Read the model definition and answer for the solid it produces. Units are mm, in the model's axes. Face numbers are marked on the shaded views. A direction names the side the tool comes from. Round coordinates to 2 decimals unless told otherwise and drop trailing zeros. Order: outer loops, then holes, each group sorted by start corner. A loop starts at its lowest first (then second) coordinate and runs counter-clockwise, first axis right, second up. Notation, with made-up numbers: (9.5, 13) - (27.5, 13) arc R21 ccw to (27.5, 41) - close; hole circle Ø8 at (-8.75, 4.5). An arc over 180 degrees is marked (long way). Put each result on its own line as item: value. Start each with the question number.
Q1. Which of the six approach directions +Z, -Z, +X, -X, +Y, -Y give full straight-line access (tool end or side, diameter ignored) to the marked faces 3 and 4?
Q2. Find the intervals of material crossed by line 1 along Y through (x, z) = (2.3, 28.5); line 2 along X through (y, z) = (0.75, 5.5); line 3 along Y through (x, z) = (1.65, 30), in increasing order. Write a range as from..to.
Q3. Section A-A on z = 15.5 is taken. Give the vertices of the cut face in (x, y), then the cut area to 3 significant figures.
Q4. For a pull along Z with two mould halves and no side action, classify the marked faces 1 and 2 as pulls with the +Z half, pulls with the -Z half, needs draft (parallel to the pull), parting line crosses it, or undercut.
Q5. Each of these flat-tipped pins is pushed along its axis until it touches: pin 1 Ø3 at (x, z) = (2, 20.5) entering from +Y; pin 2 Ø1 at (x, z) = (2.5, 16.5) entering from -Y; pin 3 Ø0.8 at (x, y) = (3.5, 1) entering from +Z. Where does it stop, or does it pass through?
Q6. Section B-B on z = 34 is taken. Give the vertices of the cut face in (x, y).
from build123d import *

# Parameters (mm, degrees)
SZKIC1_R                     = 2.5
DODANIE_WYCI_GNI_CIE1_DEPTH  = 0.31804017
SZKIC3_R                     = 2.5
DODANIE_WYCI_GNI_CIE2_DEPTH  = 0.31804017
SZKIC8_W                     = 2.5
SZKIC8_H                     = 0.31804017
SZKIC9_R                     = 2.5
DODANIE_WYCI_GNI_CIE3_DEPTH  = 0.31804017
SZKIC15_R                    = 2.5
DODANIE_WYCI_GNI_CIE4_DEPTH  = 0.31804017
SZKIC21_W                    = 2.5
SZKIC21_H                    = 0.31804017
SZKIC22_R                    = 2.5
DODANIE_WYCI_GNI_CIE5_DEPTH  = 0.31804017
SZKIC28_R                    = 2.5
DODANIE_WYCI_GNI_CIE6_DEPTH  = 0.31804017
SZKIC34_W                    = 2.5
SZKIC34_H                    = 0.31804017
DODANIE_WYCI_GNI_CIE7_DEPTH  = 0.31804017
DODANIE_WYCI_GNI_CIE8_DEPTH  = 27.657744359
DODANIE_WYCI_GNI_CIE9_DEPTH  = 0.31804017
DODANIE_WYCI_GNI_CIE10_DEPTH = 33.257744359
SZKIC54_W                    = 7.444504345
SZKIC54_H                    = 0.582583156
WYTNIJ_WYCI_GNI_CIE2_DEPTH   = 1


with BuildPart() as part:
    # Szkic1 → Dodanie-wyciągnięcie1 (new body)
    with BuildSketch(Plane.XY.offset(5)):
        with Locations((2.5, 0.25)):
            Circle(SZKIC1_R)
    extrude(amount=DODANIE_WYCI_GNI_CIE1_DEPTH)

    # Szkic3 → Dodanie-wyciągnięcie2 (add)
    with BuildSketch(Plane.XY.offset(5)):
        with Locations((2.5, -0.25)):
            Circle(SZKIC3_R)
    extrude(amount=DODANIE_WYCI_GNI_CIE2_DEPTH)

    # Szkic8 → Wycięcie-obrót2 (revolve, cut)
    with BuildSketch(Plane(origin=(0, -0.25, 0), x_dir=(1, 0, 0), z_dir=(0, 1, 0))):
        with Locations((3.75, -5.183235556)):
            Rectangle(SZKIC8_W, SZKIC8_H)
    revolve(axis=Axis((2.5, -0.25, 5.024215471), (0, 0, 1)), mode=Mode.SUBTRACT)

    # Szkic9 → Dodanie-wyciągnięcie3 (add)
    with BuildSketch(Plane.XY.offset(5.024215471)):
        with Locations(Location((2.5, 0.25, 0), (0, 0, 185.739170477))):
            Circle(SZKIC9_R)
    extrude(amount=DODANIE_WYCI_GNI_CIE3_DEPTH)

    # Szkic15 → Dodanie-wyciągnięcie4 (add)
    with BuildSketch(Plane.XY.offset(5)):
        with Locations((2.5, -0.25)):
            Circle(SZKIC15_R)
    extrude(amount=DODANIE_WYCI_GNI_CIE4_DEPTH)

    # Szkic21 → Wycięcie-obrót4 (revolve, cut)
    with BuildSketch(Plane(origin=(0, -0.25, 0), x_dir=(1, 0, 0), z_dir=(0, 1, 0))):
        with Locations((3.75, -5.183235556)):
            Rectangle(SZKIC21_W, SZKIC21_H)
    revolve(axis=Axis((2.5, -0.25, 5.024215471), (0, 0, 1)), mode=Mode.SUBTRACT)

    # Szkic22 → Dodanie-wyciągnięcie5 (add)
    with BuildSketch(Plane.XY.offset(5.024215471)):
        with Locations(Location((2.5, 0.25, 0), (0, 0, 185.739170477))):
            Circle(SZKIC22_R)
    extrude(amount=DODANIE_WYCI_GNI_CIE5_DEPTH)

    # Szkic28 → Dodanie-wyciągnięcie6 (add)
    with BuildSketch(Plane.XY.offset(5)):
        with Locations((2.5, -0.25)):
            Circle(SZKIC28_R)
    extrude(amount=DODANIE_WYCI_GNI_CIE6_DEPTH)

    # Szkic34 → Wycięcie-obrót6 (revolve, cut)
    with BuildSketch(Plane(origin=(0, -0.25, 0), x_dir=(1, 0, 0), z_dir=(0, 1, 0))):
        with Locations((3.75, -5.183235556)):
            Rectangle(SZKIC34_W, SZKIC34_H)
    revolve(axis=Axis((2.5, -0.25, 5.024215471), (0, 0, 1)), mode=Mode.SUBTRACT)

    # Szkic35 → Dodanie-wyciągnięcie7 (add)
    with BuildSketch(Plane.XY.offset(5)):
        with BuildLine():
            Line((5, 0.25), (0, 0.25))
            ThreePointArc((0, 0.25), (0.732233047, 2.017766953), (2.5, 2.75))
            ThreePointArc((2.5, 2.75), (4.267766953, 2.017766953), (5, 0.25))
        make_face()
    extrude(amount=DODANIE_WYCI_GNI_CIE7_DEPTH)

    # Szkic41 → Dodanie-wyciągnięcie8 (add)
    with BuildSketch(Plane.XY.offset(5.342255641)):
        with BuildLine():
            Line((5, 0.25), (0, 0.25))
            ThreePointArc((0, 0.25), (2.5, 2.75), (5, 0.25))
        make_face()
    extrude(amount=DODANIE_WYCI_GNI_CIE8_DEPTH)

    # Szkic42 → Dodanie-wyciągnięcie9 (add)
    with BuildSketch(Plane.XY.offset(5.024215471)):
        with BuildLine():
            Line((0, -0.25), (5, -0.25))
            ThreePointArc((5, -0.25), (4.267766953, -2.017766953), (2.5, -2.75))
            ThreePointArc((2.5, -2.75), (0.732233047, -2.017766953), (0, -0.25))
        make_face()
    extrude(amount=DODANIE_WYCI_GNI_CIE9_DEPTH)

    # Szkic43 → Dodanie-wyciągnięcie10 (add)
    with BuildSketch(Plane.XY.offset(5.342255641)):
        with BuildLine():
            Line((0, -0.25), (5, -0.25))
            ThreePointArc((5, -0.25), (2.5, -2.75), (0, -0.25))
        make_face()
    extrude(amount=DODANIE_WYCI_GNI_CIE10_DEPTH)

    # Wyciągnięcie po ścieżce1: sweep along a path in Szkic44
    with BuildLine(Plane(origin=(0, 0, 0), x_dir=(0, 0, -1), z_dir=(1, 0, 0))) as wyci_gni_cie_po_cie_ce1_path:
        Line((-5.560489768, 1.625), (0, 3.226324699))
        ThreePointArc((0, 3.226324699), (4.289893436, -0.0025), (0, -3.231324699))
        Line((0, -3.231324699), (-5.560489768, -1.63))
    # Szkic45 → Wyciągnięcie po ścieżce1 (sweep)
    with BuildSketch(Plane(origin=(0, -0.023604125, 5.269796381), x_dir=(-1, 0, 0), z_dir=(0, 0.17364817766693072, -0.984807753012208))):
        with BuildLine():
            Line((-3.646e-06, 0.226802786), (-4.999996354, 0.226802786))
            add(Edge.make_bspline(
                [(-3.646e-06, 0.226802786), (-0.004266201, 2.684617196), (-2.5, 2.684617196), (-4.995733799, 2.684617196), (-4.999996354, 0.226802786)],
                knots=[0.001707937, 0.001707937, 0.001707937, 1.570796327, 1.570796327, 3.139884716, 3.139884716, 3.139884716], degree=2, weights=[1, 0.70771037, 1, 0.70771037, 1]))
        make_face()
    sweep(path=wyci_gni_cie_po_cie_ce1_path.line)

    # Szkic54 → Wytnij-wyciągnięcie2 (cut)
    with BuildSketch(Plane(origin=(0, 0, 5), x_dir=(-1, 0, 0), z_dir=(0, 0, -1))):
        with Locations((-2.109396602, -0.0025)):
            Rectangle(SZKIC54_W, SZKIC54_H)
    extrude(amount=-WYTNIJ_WYCI_GNI_CIE2_DEPTH, mode=Mode.SUBTRACT)


solid = part.part
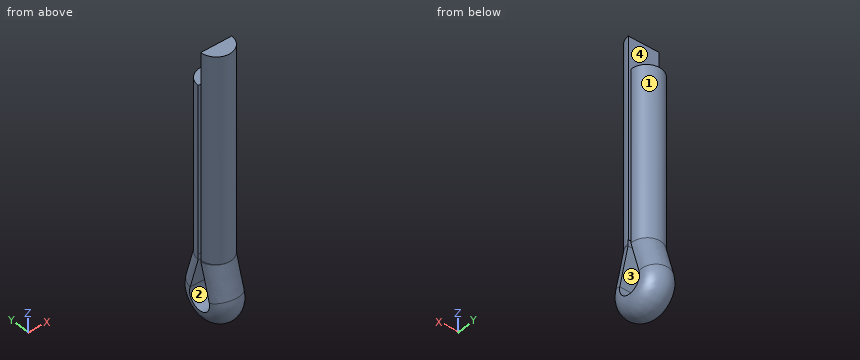
Findings:
1. face 3: +X, -X
1. face 4: +Z, +X, -X
2. line 1: -2.74..-0.25, 0.25..2.74
2. line 2: 0.05..4.95
2. line 3: -2.6..-0.25, 0.25..2.6
3. outline: (0, -0.25) arc R2.5 ccw to (5, -0.25) - close; (0, 0.25) - (5, 0.25) arc R2.5 ccw to start
3. area: 19.6 mm2
4. face 1: needs draft
4. face 2: undercut
5. pin 1: y = 2.75
5. pin 2: y = -2.75
5. pin 3: z = 33
6. outline: (0, -0.25) arc R2.5 ccw to (5, -0.25) - close
